Design review of the part built by this model. Coordinates are the model's own, in mm. A direction names the side the tool comes from. Give positions to 0.01 mm unless a question says otherwise; leave off trailing zeros. Loops run counter-clockwise (first coordinate to the right, second up) from the corner with the lowest first, then second, coordinate; pieces in that order, holes last. Notation, with made-up numbers: (60, 44.5) -> (83, 44.5) arc R29 cw to (83, 73.5) -> close; hole circle Ø6 at (-38, -1). An arc over 180 degrees is marked (long way). Answer as CSV lines item,"result".
from build123d import *

# Parameters (mm, degrees)
F0_W        = 87.937258184
F0_H        = 36.5022588521
F0_R        = 9.2048285636
F1_DEPTH    = 25.4
F2_T1_DEPTH = 113.337258184
F2_T3_DEPTH = 61.9022588521
F3_DEPTH    = 45.72


# Not quite as in the source:
# - a fillet or chamfer that OpenCascade refuses, or shapes differently, is made with other operations: its cross-section is extruded or revolved along the edge and cut away or added


with BuildPart() as f1:
    # F0 (on Top) → F1 (new body)
    with BuildSketch(Plane.XY):
        with Locations((-1.4748387039, -2.3044357076)):
            Rectangle(F0_W, F0_H)
        with Locations((-11.1534688622, 4.1479840875)):
            Circle(F0_R, mode=Mode.SUBTRACT)
    extrude(amount=F1_DEPTH)

    # F2: fillet of radius 5.08 on 6 edges, made by hand

    # F2_s2 → F2_t1 (cut)
    with BuildSketch(Plane.YZ.offset(-58.1434677958)):
        with BuildLine():
            ThreePointArc((-20.5555651337, 20.32), (-19.0676675821, 23.9121024484), (-15.4755651337, 25.4))
            Line((-15.4755651337, 25.4), (-20.5555651337, 25.4))
            Line((-20.5555651337, 25.4), (-20.5555651337, 20.32))
        make_face()
        with BuildLine():
            ThreePointArc((15.9466937184, 20.32), (14.4587961669, 23.9121024484), (10.8666937184, 25.4))
            Line((10.8666937184, 25.4), (15.9466937184, 25.4))
            Line((15.9466937184, 25.4), (15.9466937184, 20.32))
        make_face()
        with BuildLine():
            ThreePointArc((-20.5555651337, 5.08), (-19.0676675821, 1.4878975516), (-15.4755651337, 0))
            Line((-15.4755651337, 0), (-20.5555651337, 0))
            Line((-20.5555651337, 0), (-20.5555651337, 5.08))
        make_face()
    extrude(amount=F2_T1_DEPTH, mode=Mode.SUBTRACT)

    # F2_s4 → F2_t3 (cut)
    with BuildSketch(Plane.XZ.offset(-28.6466937184)):
        with BuildLine():
            ThreePointArc((-45.4434677958, 20.32), (-43.9555702443, 23.9121024484), (-40.3634677958, 25.4))
            Line((-40.3634677958, 25.4), (-45.4434677958, 25.4))
            Line((-45.4434677958, 25.4), (-45.4434677958, 20.32))
        make_face()
        with BuildLine():
            ThreePointArc((42.4937903881, 20.32), (41.0058928365, 23.9121024484), (37.4137903881, 25.4))
            Line((37.4137903881, 25.4), (42.4937903881, 25.4))
            Line((42.4937903881, 25.4), (42.4937903881, 20.32))
        make_face()
        with BuildLine():
            ThreePointArc((42.4937903881, 5.08), (41.0058928365, 1.4878975516), (37.4137903881, 0))
            Line((37.4137903881, 0), (42.4937903881, 0))
            Line((42.4937903881, 0), (42.4937903881, 5.08))
        make_face()
    extrude(amount=F2_T3_DEPTH, mode=Mode.SUBTRACT)

    # F3 (add): a face of the model
    f3_faces = [f1.faces().sort_by_distance(p)[0] for p in [
        (-0.1621567776, -3.0875160288, 25.4),
    ]]
    extrude(f3_faces, amount=F3_DEPTH)


solid = f1.part
Q1. We need section C-C, the plane z = 33. State the section outline as (x, y) points.
Filled sheet:
outline,"(-40.36, -15.48) -> (37.41, -15.48) -> (37.41, 10.87) -> (-4.86, 10.87) arc R9.2 cw (long way) to (-17.45, 10.87) -> (-40.36, 10.87) -> close"
Q2. We need section D-D, the plane y = -14. State the section outline as (x, z) points.
Filled sheet:
outline,"(-45.44, 0) -> (37.41, 0) arc R5.08 ccw to (42.49, 5.08) -> (42.49, 20.32) arc R5.08 ccw to (37.41, 25.4) -> (37.41, 71.12) -> (-40.36, 71.12) -> (-40.36, 25.4) arc R5.08 ccw to (-45.44, 20.32) -> close"
Q3. We need section B-B, the plane x = 12. State the section outline as (y, z) points, and give its area (3 significant figures).
Filled sheet:
outline,"(-20.56, 5.08) arc R5.08 ccw to (-15.48, 0) -> (15.95, 0) -> (15.95, 20.32) arc R5.08 ccw to (10.87, 25.4) -> (10.87, 71.12) -> (-15.48, 71.12) -> (-15.48, 25.4) arc R5.08 ccw to (-20.56, 20.32) -> close"
area,"2,110 mm^2"
Q4. For faces 1 (the flat face through (-40.363, -2, 48)), 2 (the flat face through (-2, -15.476, 48)), 3 (the flat face through (16, 10.867, 48)), 4 (the flat face through (37.414, -2, 48)), list the 3-axis set-ups (+Z, -Z, +X, -X, +Y, -Y) from which the entire face can be reached by the end or side of a thin tool; tool diameter is ignored.
Filled sheet:
face 1,"+Z, -X, +Y, -Y"
face 2,"+Z, +X, -X, -Y"
face 3,"+Z, +X, -X, +Y"
face 4,"+Z, +X, +Y, -Y"
Q5. The part is to be moulded in two halves that separate along Y. For faces 5 (the cylindrical face through (-2.73, 0.44, 35.06)), 6 (the flat face through (-2, -20.556, 13)), 7 (the cylindrical face through (41.05, -2.05, 23.87)), say which applies: pulls with the +Y half, pulls with the -Y half, needs draft (parallel to the pull), parting line crosses it, or undercut.
Filled sheet:
face 5,"undercut"
face 6,"pulls with the -Y half"
face 7,"needs draft"
Q6. Clearance check with flat-ended pins moving along their axes: pin 1 Ø8 at (y, z) = (8.5, 36) entering from -X; pin 2 Ø12 at (y, z) = (1.5, 34) entering from +X; pin 3 Ø1.5 at (x, z) = (-21, 39.5) entering from +Y; pin 4 Ø12 at (x, y) = (20.5, -8.5) entering from -Z. State where each tip first meets the part, or that it passes through.
Filled sheet:
pin 1,"stops at x = -40.36"
pin 2,"stops at x = 37.41"
pin 3,"stops at y = 10.87"
pin 4,"stops at z = 0"
Q7. To check wall thickness, follow probe 1 along X at (y, z) = (3.5, 13); probe 2 along X at (y, z) = (-12.5, 50.5); probe 3 along Y at (x, z) = (28.5, 37). State the ranges of each line that lie inside material, in increasing order. Write a range as from..to.
Filled sheet:
probe 1,"x = -45.44..-20.34, -1.97..42.49"
probe 2,"x = -40.36..37.41"
probe 3,"y = -15.48..10.87"
Q8. We need section A-A, the plane y = 8.5. State the section outline as (x, z) points, and give its area (3 significant figures).
Filled sheet:
outline,"(-45.44, 0) -> (-19.26, 0) -> (-19.26, 71.12) -> (-40.36, 71.12) -> (-40.36, 25.4) arc R5.08 ccw to (-45.44, 20.32) -> close; (-3.04, 0) -> (37.41, 0) arc R5.08 ccw to (42.49, 5.08) -> (42.49, 20.32) arc R5.08 ccw to (37.41, 25.4) -> (37.41, 71.12) -> (-3.04, 71.12) -> close"
area,"4,620 mm^2"
